The model under review builds one solid part; all positions refer to its coordinate system, in mm. Face numbers are marked on the shaded views. A direction names the side the tool comes from. Round coordinates to 2 decimals unless told otherwise and drop trailing zeros. Write each loop counter-clockwise with the first axis right and the second up, starting at its lowest first coordinate (ties: lowest second). Pieces come first, ordered by that corner, then holes.
Item 1: Machinability: for the marked faces 1 and 2, which of the approach directions +Z, -Z, +X, -X, +Y, -Y give a long, thin tool a straight path to every point of the face, cutting with its end or side? Answer none if there is none.
Item 2: Add section A-A (y = -6.75). Give the boundary of the cut face in (x, z).
Item 3: To check wall thickness, follow L1, parallel to Z at x = 0, y = 0.75 (3 decimals); L2, parallel to X at y = -3.25, z = 11.5; L3, parallel to Z at x = -3.25, y = -3.75. State the ranges of each line that lie inside material, in increasing order.
Item 4: Clearance check with flat-ended pins moving along their axes: pin 1 Ø12.5 at (x, z) = (-2.5, 35.5) entering from -Y; pin 2 Ø12 at (x, z) = (-5.5, 53.5) entering from -Y; pin 3 Ø0.6 at (y, z) = (0.5, 30.5) entering from -X. State where each tip first meets the part, or that it passes through.
Item 5: Add section C-C (x = 0). Give the boundary of the cut face in (y, z) (3 decimals), plus the area to 3 significant figures.
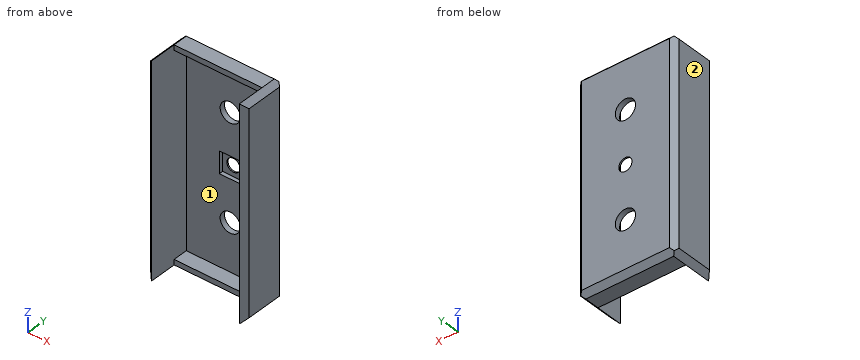
```python
from build123d import *

# Parameters (mm, degrees)
F1_DEPTH  = 59.8
F2_R      = 2.875
F2_R_2    = 1.875
F3_DEPTH  = 25
F4_W      = 25
F4_H      = 4.2
F5_DEPTH  = 1.5
F6_W      = 25
F6_H      = 4.2
F7_DEPTH  = 1.5
F8_SIZE   = 1.5
F9_SIZE   = 1.5
F11_DEPTH = 1.1
F12_SIZE  = 1.49999


# Not quite as in the source:
# - a fillet or chamfer is up to 0.001 mm smaller than in the source, because OpenCascade refuses the exact size


with BuildPart() as f1:
    # F0 (on Top) → F1 (new body)
    with BuildSketch(Plane.XY):
        Polygon((-12.5, 0), (0, 0), (0, 1.5), (-12.5, 1.5), (-14, 1.5), (-14, 0), (-14, -12), (-12.5, -12), align=None)
        Polygon((0, 1.5), (0, 0), (12.5, 0), (12.5, -12), (14, -12), (14, 0), (14, 1.5), (12.5, 1.5), align=None)
    extrude(amount=F1_DEPTH)

    # F2 (on face) → F3 (cut)
    with BuildSketch(Plane(origin=(0, 1.5, 0), x_dir=(-1, 0, 0), z_dir=(0, 1, 0))):
        with Locations((0, 44.85)):
            Circle(F2_R)
        with Locations((0, 29.9)):
            Circle(F2_R_2)
        with Locations((0, 14.95)):
            Circle(F2_R)
    extrude(amount=-F3_DEPTH, mode=Mode.SUBTRACT)

    # F4 (on face) → F5 (join)
    with BuildSketch(Plane.XY.offset(59.8)):
        with Locations((0, -2.1)):
            Rectangle(F4_W, F4_H)
    extrude(amount=-F5_DEPTH)

    # F6 (on face) → F7 (join)
    with BuildSketch(Plane(origin=(0, 0, 0), x_dir=(1, 0, 0), z_dir=(0, 0, -1))):
        with Locations((0, 2.1)):
            Rectangle(F6_W, F6_H)
    extrude(amount=-F7_DEPTH)

    # F8
    f8_edges = [f1.edges().sort_by_distance(p)[0] for p in [
        (14, 1.5, 29.9),
        (-14, 1.5, 29.9),
        (0, 1.5, 0),
        (0, 1.5, 59.8),
    ]]
    chamfer(f8_edges, length=F8_SIZE)

    # F9
    f9_edges = [f1.edges().sort_by_distance(p)[0] for p in [
        (-14, -6, 0),
        (14, -6, 0),
        (-14, -6, 59.8),
        (14, -6, 59.8),
    ]]
    chamfer(f9_edges, length=F9_SIZE)

    # F10 (on face) → F11 (cut)
    with BuildSketch(Plane.XZ):
        Polygon((3.1, 33), (0, 33), (-3.1, 33), (-3.1, 26.8), (0, 26.8), (3.1, 26.8), (3.1, 29.9), align=None)
    extrude(amount=-F11_DEPTH, mode=Mode.SUBTRACT)

    # F12 (size 1.5 in the source; OpenCascade refuses exactly that, so slightly less here)
    f12_edges = [f1.edges().sort_by_distance(p)[0] for p in [
        (-14, -12, 29.9),
        (14, -12, 29.9),
    ]]
    chamfer(f12_edges, length=F12_SIZE)


solid = f1.part
```
Numbers:
1. face 1: -Y
1. face 2: +Z, -Z, -X, +Y, -Y
2. outline: (-14, 1.5) - (-12.5, 0) - (-12.5, 59.8) - (-14, 58.3) - close; (12.5, 0) - (14, 1.5) - (14, 58.3) - (12.5, 59.8) - close
3. L1: z = 0.75 to 12.075, 17.825 to 26.8, 33 to 41.975, 47.725 to 59.05
3. L2: x = -14 to -12.5, 12.5 to 14
3. L3: z = 0 to 1.5, 58.3 to 59.8
4. pin 1: stops at y = 0
4. pin 2: stops at y = -4.2
4. pin 3: stops at x = -13.8
5. outline: (-4.2, 0) - (0, 0) - (1.5, 1.5) - (1.5, 12.075) - (0, 12.075) - (0, 1.5) - (-4.2, 1.5) - close; (-4.2, 58.3) - (0, 58.3) - (0, 47.725) - (1.5, 47.725) - (1.5, 58.3) - (0, 59.8) - (-4.2, 59.8) - close; (0, 17.825) - (1.5, 17.825) - (1.5, 28.025) - (1.1, 28.025) - (1.1, 26.8) - (0, 26.8) - close; (0, 33) - (1.1, 33) - (1.1, 31.775) - (1.5, 31.775) - (1.5, 41.975) - (0, 41.975) - close
5. area: 74.5 mm2
